from build123d import *

# Parameters (mm, degrees)
CROSSRECESS_DEPTH = 2.325
DRAFT9_ANGLE      = 30
FILLET5_R         = 0.3
LPATTERN10_COUNT  = 7
LPATTERN10_PITCH  = 0.8118


with BuildPart() as part:
    # Sketch1 → Base (revolve)
    with BuildSketch(Plane.XY):
        Polygon((10, 4), (7.15, 4), (4.65, 4), (0.965, 7.685), (0, 7.685), (0, 0), (10, 0), align=None)
    revolve(axis=Axis((4.515812911, 0, 0), (-1, 0, 0)))

    # Sketch6 → CrossRecess (cut)
    with BuildSketch(Plane(origin=(0, 0, 0), x_dir=(0, 0, -1), z_dir=(1, 0, 0))):
        Polygon((0.89, 0.89), (0.89, 4.45), (-0.89, 4.45), (-0.89, 0.89), (-4.45, 0.89), (-4.45, -0.89), (-0.89, -0.89), (-0.89, -4.45), (0.89, -4.45), (0.89, -0.89), (4.45, -0.89), (4.45, 0.89), align=None)
    extrude(amount=CROSSRECESS_DEPTH, mode=Mode.SUBTRACT)

    # Draft9
    draft9_faces = [part.faces().sort_by_distance(p)[0] for p in [
        (1.1625, 4.45, 0),
        (1.1625, 0, 4.45),
        (1.1625, -4.45, 0),
        (1.1625, 0, -4.45),
    ]]
    draft(draft9_faces, Plane(origin=(0, 7.685, 0), x_dir=(0, 0, -1), z_dir=(-1, 0, 0)), DRAFT9_ANGLE)

    # Fillet5
    fillet5_edges = [part.edges().sort_by_distance(p)[0] for p in [
        (1.1625, 0.89, 0.89),
        (1.1625, -0.89, 0.89),
        (1.1625, -0.89, -0.89),
        (1.1625, 0.89, -0.89),
    ]]
    fillet(fillet5_edges, radius=FILLET5_R)

    # Sketch9 → Cut-Revolve10 (revolve, cut)
    with BuildSketch(Plane.XY):
        Polygon((10, 3.414133814), (10.33825, 4), (10.33825, 4.6765), (9.66175, 4.6765), (9.66175, 4), align=None)
    cut_revolve10 = revolve(axis=Axis((0, 0, 0), (1, 0, 0)), mode=Mode.SUBTRACT)

    # LPattern10: Cut-Revolve10 ×7
    with Locations(*[(-i * LPATTERN10_PITCH, 0, 0) for i in range(1, LPATTERN10_COUNT)]):
        add(cut_revolve10, mode=Mode.SUBTRACT)


solid = part.part
Geometry: final body of the model. Coordinates: model frame, mm. A direction names the side the tool comes from. Give positions to 0.01 mm unless a question says otherwise; leave off trailing zeros. Write each loop counter-clockwise with the first axis right and the second up, starting at its lowest first coordinate (ties: lowest second). Pieces come first, ordered by that corner, then holes. Notation, with made-up numbers: M 3.25,61 L 42.25,61 A16 cw 42.25,73 Z; hole C 50,59.25 d10. An arc over 180 degrees is marked long. Answer in a Markdown table with one row per item. Add a question column.
(1) Ray query, line 1 (Z direction, x = 1.25, y = -1); line 2 (Y direction, x = 2, z = -1.25); line 3 (Y direction, x = 1.5, z = -2). Return the intervals inside material, ascending.
(2) Section A-A on x = 1.75. Return loops of the section in (y, z).
(3) First-contact query: pin 1 (0.7 mm diameter, centred on x = 1, y = -2, fed in from -Z); pin 2 (0.7 mm diameter, centred on x = 1, z = -3, fed in from -Y); pin 3 (1.5 mm diameter, centred on x = 8, z = -1.5, fed in from -Y). Flat tips, straight axial feed; report the tip coordinate or a pass-through.
(4) Reachability of faces 1 (the conical face through (4.42, -0.92, 4.13)), 2 (the flat face through (1, -2, 0.89)) from +Z, -Z, +X, -X, +Y, -Y: full face, straight path, thin tool, end or side. Return the list, or none.
Result set:
| question | item | result |
|---|---|---|
| 1 | line 1 | z = -7.33 to -0.96, 0.96 to 7.33 |
| 1 | line 2 | y = -6.53 to -0.89, 0.89 to 6.53 |
| 1 | line 3 | y = -6.86 to -0.89, 0.89 to 6.86 |
| 2 | outline | C 0,0 d13.8; hole M -3.44,-0.89 L -1.19,-0.89 A0.3 cw -0.89,-1.19 L -0.89,-3.44 L 0.89,-3.44 L 0.89,-1.19 A0.3 cw 1.19,-0.89 L 3.44,-0.89 L 3.44,0.89 L 1.19,0.89 A0.3 cw 0.89,1.19 L 0.89,3.44 L -0.89,3.44 L -0.89,1.19 A0.3 cw -1.19,0.89 L -3.44,0.89 Z |
| 3 | pin 1 | stops at z = -7.51 |
| 3 | pin 2 | stops at y = -7.21 |
| 3 | pin 3 | stops at y = -3.93 |
| 4 | face 1 | +X |
| 4 | face 2 | -X |
